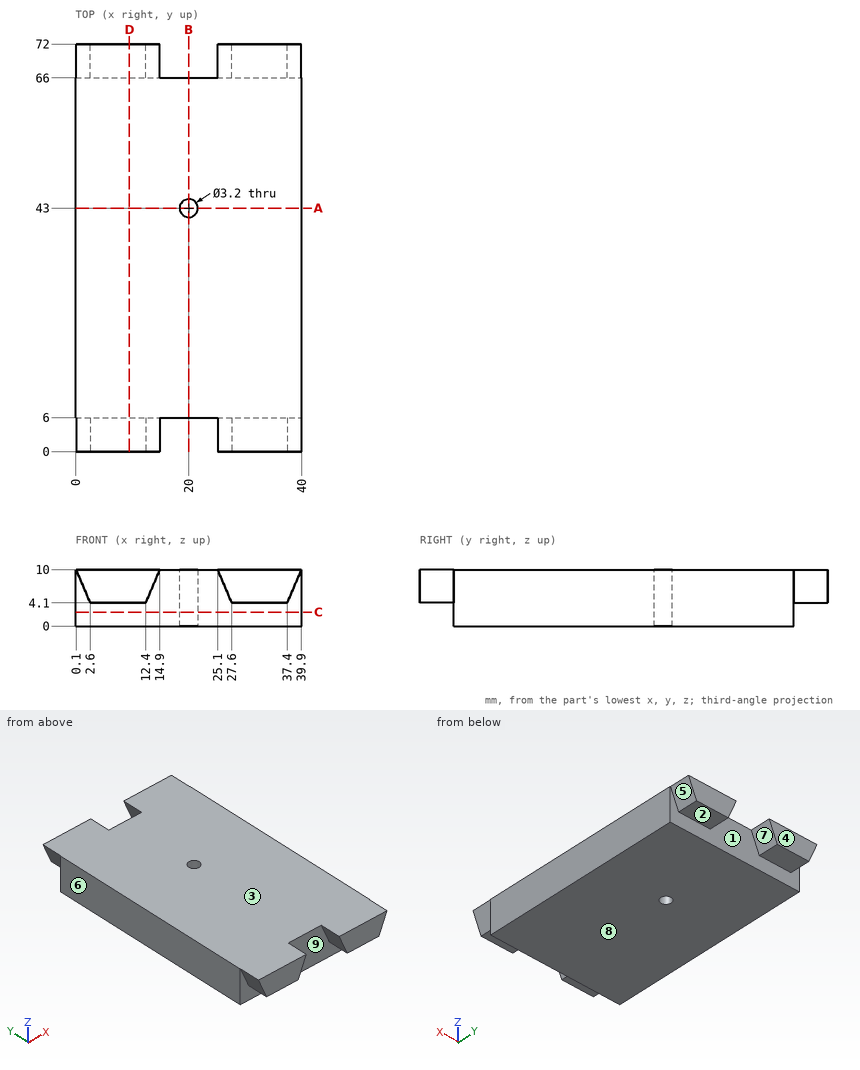
Print and shaded views of the part. All mm, measured from the part's lowest x, y and z. A direction names the side the tool comes from. Give positions to 0.01 mm unless a question says otherwise; leave off trailing zeros. Write each loop counter-clockwise with the first axis right and the second up, starting at its lowest first coordinate (ties: lowest second). Pieces come first, ordered by that corner, then holes. Notation, with made-up numbers: M 26,-33.5 L 67,-33.5 A23 cw 67,-12.5 Z; hole C 42,-27.5 d10. An arc over 180 degrees is marked long. Use a Markdown table: item, result.
1) Drill centre lines: line 1 (Y direction, x = 20, z = 7); line 2 (Y direction, x = 36.5, z = 2.5); line 3 (X direction, y = 42, z = 4). Where is each one in solid material? Low to high. Write a range as from..to.
Responses:
| item | result |
|---|---|
| line 1 | y = 6..41.4, 44.6..66 |
| line 2 | y = 6..66 |
| line 3 | x = 0..18.75, 21.25..40 |
2) Cut at A-A (y = 43). List the corners of the cut face in (x, z).
Responses:
| item | result |
|---|---|
| outline | M 0,0 L 18.4,0 L 18.4,10 L 0,10 Z; M 21.6,0 L 40,0 L 40,10 L 21.6,10 Z |
3) Pull direction X, two halves, no side cores. Call the marked faces 6, 7, 8 and 9: +X half, -X half, draft (parallel to the pull), parting line (faces both ways), or undercut.
Responses:
| item | result |
|---|---|
| face 6 | -X half |
| face 7 | undercut |
| face 8 | draft |
| face 9 | undercut |
4) Pin check, flat tips, straight feed: pin 1 (5 mm diameter, centred on y = 64.5, z = 7.5, fed in from -X); pin 2 (6.5 mm diameter, centred on x = 32, y = 2, fed in from -Z); pin 3 (4 mm diameter, centred on x = 23.5, z = 6.5, fed in from +Y). Stop position of each tip, or through.
Responses:
| item | result |
|---|---|
| pin 1 | stops at x = 0 |
| pin 2 | stops at z = 4.1 |
| pin 3 | stops at y = 66 |
5) Cut at B-B (x = 20). List the corners of the cut face in (y, z), and give its area (3 significant figures).
Responses:
| item | result |
|---|---|
| outline | M 6,0 L 41.4,0 L 41.4,10 L 6,10 Z; M 44.6,0 L 66,0 L 66,10 L 44.6,10 Z |
| area | 568 mm2 |
6) Cut at D-D (x = 9.5). List the corners of the cut face in (y, z), and give its area (3 significant figures).
Responses:
| item | result |
|---|---|
| outline | M 0,4.1 L 6,4.1 L 6,0 L 66,0 L 66,4.1 L 72,4.1 L 72,10 L 0,10 Z |
| area | 671 mm2 |
7) Tool access for the marked faces 1, 2, 3, 4 and 5: list every direction of +Z, -Z, +X, -X, +Y, -Y with a clear straight run to the whole face (end or side of a thin tool).
Responses:
| item | result |
|---|---|
| face 1 | -Z, +Y |
| face 2 | -Z, +X, -X, +Y |
| face 3 | +Z, +X, -X, +Y, -Y |
| face 4 | +Z, -Z, +X, -X, +Y |
| face 5 | -Z, +X, +Y |
8) Cut at C-C (z = 2.5). List the corners of the cut face in (x, y), and give its area (3 significant figures).
Responses:
| item | result |
|---|---|
| outline | M 0,6 L 40,6 L 40,66 L 0,66 Z; hole C 20,43 d3.2 |
| area | 2,390 mm2 |
